Source: CAD feature listing. Evaluate the final solid. Frame: model axes, mm. A direction names the side the tool comes from. Give positions to 0.01 mm unless a question says otherwise; leave off trailing zeros. Write each loop counter-clockwise with the first axis right and the second up, starting at its lowest first coordinate (ties: lowest second). Pieces come first, ordered by that corner, then holes. Notation, with made-up numbers: (15, -28) - (74, -28) arc R27 ccw to (74, 2) - close; hole circle Ø11 at (-6.5, 31). An arc over 180 degrees is marked (long way). One line per question, with ' | ' between items. Start each with the question number.
(1) Pin query (flat end, axial travel): pin 1 (1.5 mm diameter, centred on x = -11, y = -25.5, fed in from +Z); pin 2 (2 mm diameter, centred on y = 5, z = 2.5, fed in from +X); pin 3 (2 mm diameter, centred on x = -17.5, z = -9, fed in from +Y). Return the tip coordinate at first contact, or that it passes through.
(2) Access query for faces 1 (the cylindrical face through (36.4, -43.4, 5.4)), 2 (the flat face through (55.04, -52.11, 5.24)), 3 (the cylindrical face through (-10.33, 27.48, 8.1)), 4 (the flat face through (35.6, 17.5, 5.2)). Directions: +Z, -Z, +X, -X, +Y, -Y. A direction counts if a zero-diameter tool reaches every point of the face in a straight line with its end or side. Return the directions, or none.
(3) Section B-B, the plane y = 37.5. Return loops of the section in (x, z), plus the area to 3 significant figures.
(4) Section A-A, the plane z = -26. Return loops of the section in (x, y).
(5) Draft query along Y for faces 5 (the flat face through (56.35, 3.54, 5.24)), 6 (the cylindrical face through (76.888, 4.301, 5.34)), 7 (the flat face through (-15.44, -58.41, 5.24)), 8 (the flat face through (-35.263, 47.32, 5.24)). Return one class per face: +Y half, -Y half, draft (parallel to the pull), parting line (faces both ways), or undercut.
(6) Section C-C, the plane z = -10. Return loops of the section in (x, y).
(7) Ray query, line 1 (Y direction, x = -10, z = 7); line 2 (Z direction, x = 19, y = -41.5); line 3 (Y direction, x = -10, z = 8.65). Return the intervals inside material, ascending. Write a range as [from, to].
```python
from build123d import *

# Parameters (mm, degrees)
RESSALTO_EXTRUS_O1_DEPTH = 10
RESSALTO_EXTRUS_O1_DRAFT = -9
ESBO_O2_R                = 23
RESSALTO_EXTRUS_O2_DEPTH = 30
RESSALTO_EXTRUS_O2_DRAFT = -9
FILETE1_R                = 10
FILETE2_R                = 2.5
ESCALA1_SCALE            = 1.05
ESBO_O3_R                = 2.5
CORTE_EXTRUS_O1_DEPTH    = 5


with BuildPart() as part:
    # Esboço1 → Ressalto-extrusão1 (with draft: the straight prism first)
    with BuildSketch(Plane.XY):
        Polygon((-22.781745931, 55), (-44.375431078, 33.406314852), (-44.375431078, -33.406314852), (-22.781745931, -55), (-10.825814677, -55), (32.742040246, -49), (72.742040246, -49), (72.742040246, -43), (32.742040246, -43), (32.742040246, 4), (72.742040246, 4), (72.742040246, 10), (32.742040246, 10), (32.742040246, 20), (-10.825814677, 55), align=None)
    extrude(amount=RESSALTO_EXTRUS_O1_DEPTH)
    # Ressalto-extrusão1: the draft: its side faces are tilted about the plane it starts from
    ressalto_extrus_o1_sides = [part.faces().sort_by_distance(p)[0] for p in [
        (-33.578588504, 44.203157426, 5),
        (-44.375431078, 0, 5),
        (-33.578588504, -44.203157426, 5),
        (-16.803780304, -55, 5),
        (10.958112785, -52, 5),
        (52.742040246, -49, 5),
        (72.742040246, -46, 5),
        (52.742040246, -43, 5),
        (32.742040246, -19.5, 5),
        (52.742040246, 4, 5),
        (72.742040246, 7, 5),
        (52.742040246, 10, 5),
        (32.742040246, 15, 5),
        (10.958112785, 37.5, 5),
        (-16.803780304, 55, 5),
    ]]
    draft(ressalto_extrus_o1_sides, Plane.XY, RESSALTO_EXTRUS_O1_DRAFT)


with BuildPart() as ressalto_extrus_o2_tool:
    # Esboço2 → Ressalto-extrusão2 (with draft: the straight prism first)
    with BuildSketch(Plane.XY):
        with Locations((-20, 0)):
            Circle(ESBO_O2_R)
    extrude(amount=-RESSALTO_EXTRUS_O2_DEPTH)
    # Ressalto-extrusão2: the draft: its side faces are tilted about the plane it starts from
    ressalto_extrus_o2_sides = [ressalto_extrus_o2_tool.faces().sort_by_distance(p)[0] for p in [
        (-43, 0, -15),
    ]]
    draft(ressalto_extrus_o2_sides, Plane.XY, RESSALTO_EXTRUS_O2_DRAFT)


with BuildPart() as part_1:
    add(part.part)

    # Ressalto-extrusão2: add ressalto_extrus_o2_tool
    add(ressalto_extrus_o2_tool.part)

    # Filete1
    filete1_edges = [part_1.edges().sort_by_distance(p)[0] for p in [
        (-23.109770847, -55.791922202, 5),
    ]]
    fillet(filete1_edges, radius=FILETE1_R)

    # Filete2
    filete2_edges = [part_1.edges().sort_by_distance(p)[0] for p in [
        (33.533962448, 10.791922202, 5),
        (73.533962448, 10.791922202, 5),
        (73.533962448, 3.208077798, 5),
        (33.533962448, 3.208077798, 5),
        (33.533962448, -42.208077798, 5),
        (73.533962448, -42.208077798, 5),
        (73.533962448, -49.791922202, 5),
    ]]
    fillet(filete2_edges, radius=FILETE2_R)


with BuildPart() as part_2:
    # Escala1: scaled about (-8.171649515, -3.224100795, -1.267383115)
    add(part_1.part.scale(ESCALA1_SCALE).moved(Location((0.408582476, 0.16120504, 0.063369156))))

    # Esboço3 → Corte-extrusão1 (cut)
    with BuildSketch(Plane.XY.offset(10.563369297)):
        with Locations((-10, 25)):
            Circle(ESBO_O3_R)
        with Locations((-10, -25)):
            Circle(ESBO_O3_R)
    extrude(amount=-CORTE_EXTRUS_O1_DEPTH, mode=Mode.SUBTRACT)


solid = part_2.part
```
Check sheet entries:
1) pin 1: z = 5.56 | pin 2: x = 77.18 | pin 3: y = 22.87
2) face 1: -Z, +X | face 2: -Z, +X, -Y | face 3: +Z | face 4: -Z, +X, +Y
3) outline: (-46.28, 10.56) - (-43.92, 0.06) - (14.45, 0.06) - (17.1, 10.56) - close | area: 639 mm²
4) outline: circle Ø40.04 at (-20.59, 0.16)
5) face 5: undercut | face 6: undercut | face 7: -Y half | face 8: +Y half
6) outline: circle Ø45.11 at (-20.59, 0.16)
7) line 1: [-58.57, -27.5], [-22.5, 22.5], [27.5, 58.55] | line 2: [0.06, 10.56] | line 3: [-58.83, -27.5], [-22.5, 22.5], [27.5, 58.89]
